For this review, take the finished solid that the model builds, in its own axes (mm). A direction names the side the tool comes from. Round coordinates to 2 decimals unless told otherwise and drop trailing zeros. Write each loop counter-clockwise with the first axis right and the second up, starting at its lowest first coordinate (ties: lowest second). Pieces come first, ordered by that corner, then holes. Notation, with made-up numbers: M 32.25,18 L 66.25,18 A4 cw 66.25,22 Z; hole C 64,-20.5 d5. An arc over 180 degrees is marked long. Answer in a Markdown table with one row per item.
```python
from build123d import *

# Parameters (mm, degrees)
SKETCH_1_W          = 50
SKETCH_1_H          = 20
EXTRUDE_1_DEPTH     = 2
SKETCH_2_R          = 3
EXTRUDE_2_DEPTH     = 2
EXTRUDE_START       = -2
SKETCH_3_R          = 3
EXTRUDE_3_DEPTH     = 2
SKETCH_4_R          = 1.5
CUT_EXTRUDE_1_DEPTH = 2


with BuildPart() as part:
    # 草图1 → 凸台-拉伸1 (new body)
    with BuildSketch(Plane(origin=(0, 0, 0), x_dir=(1, 0, 0), z_dir=(0, 1, 0))):
        Rectangle(SKETCH_1_W, SKETCH_1_H)
    extrude(amount=EXTRUDE_1_DEPTH)

    # 草图2 → 凸台-拉伸2 (add)
    with BuildSketch(Plane.ZY.offset(25)):
        with BuildLine():
            Line((-10, 2), (10, 2))
            Line((10, 2), (10, -18.1))
            ThreePointArc((10, -18.1), (7.100357134, -25.100357134), (0.1, -28))
            Line((0.1, -28), (-0.1, -28))
            ThreePointArc((-0.1, -28), (-7.100357134, -25.100357134), (-10, -18.1))
            Line((-10, -18.1), (-10, 2))
        make_face()
        with Locations((0, -18.1)):
            Circle(SKETCH_2_R, mode=Mode.SUBTRACT)
    extrude(amount=-EXTRUDE_2_DEPTH)

    # 草图3 → 凸台-拉伸3 (add)
    with BuildSketch(Plane(origin=(25, 0, 0), x_dir=(0, 0, -1), z_dir=(1, 0, 0)).offset(EXTRUDE_START)):
        with BuildLine():
            Line((-10, 2), (10, 2))
            Line((10, 2), (10, -18.1))
            ThreePointArc((10, -18.1), (7.100357134, -25.100357134), (0.1, -28))
            Line((0.1, -28), (-0.1, -28))
            ThreePointArc((-0.1, -28), (-7.100357134, -25.100357134), (-10, -18.1))
            Line((-10, -18.1), (-10, 2))
        make_face()
        with Locations(Location((0, -18.1, 0), (0, 0, 180))):
            Circle(SKETCH_3_R, mode=Mode.SUBTRACT)
    extrude(amount=EXTRUDE_3_DEPTH)

    # 草图4 → 切除-拉伸1 (cut)
    with BuildSketch(Plane(origin=(0, 2, 0), x_dir=(1, 0, 0), z_dir=(0, 1, 0))):
        with Locations(Location((0, 5, 0), (0, 0, 270))):
            Circle(SKETCH_4_R)
        with Locations(Location((5, 0, 0), (0, 0, 270))):
            Circle(SKETCH_4_R)
        with Locations(Location((0, -5, 0), (0, 0, 270))):
            Circle(SKETCH_4_R)
        with Locations(Location((-5, 0, 0), (0, 0, 270))):
            Circle(SKETCH_4_R)
    extrude(amount=-CUT_EXTRUDE_1_DEPTH, mode=Mode.SUBTRACT)


solid = part.part
```
Q1. Mouldability with a two-part tool opening along Z and no side actions: class faces 1 (the face through (25, -13, 0)), 2 (the face through (-24, -25, 7.2)), 3 (the face through (-3.513, 1.014, -0.195)) as +Z half, -Z half, draft (parallel to the pull), parting line (faces both ways), or undercut.
Found:
| item | result |
|---|---|
| face 1 | draft |
| face 2 | +Z half |
| face 3 | undercut |
Q2. Machinability: for faces 4 (the face through (0, 2, 0)), 5 (the face through (0, 0, 0)), which of the approach directions +Z, -Z, +X, -X, +Y, -Y give a long, thin tool a straight path to every point of the face, cutting with its end or side? Answer none if there is none.
Found:
| item | result |
|---|---|
| face 4 | +Z, -Z, +X, -X, +Y |
| face 5 | +Z, -Z, -Y |
Q3. Take a section at C-C (z = 6). State the section outline as (x, y) points, then the cut area to 3 significant figures.
Found:
| item | result |
|---|---|
| outline | M -25,-26.05 L -23,-26.05 L -23,0 L -1.12,0 L -1.12,2 L -25,2 Z; M 1.12,0 L 23,0 L 23,-26.05 L 25,-26.05 L 25,2 L 1.12,2 Z |
| area | 200 mm² |
Q4. For probe 1 along X at (y, z) = (1.1, 0); probe 2 along Z at (x, y) = (24.45, -18.1); probe 3 along X at (y, z) = (-13.75, -1), list the stretches that pass through material, from the lowest coordinate up.
Found:
| item | result |
|---|---|
| probe 1 | -25 to -6.5, -3.5 to 3.5, 6.5 to 25 |
| probe 2 | -10 to -3, 3 to 10 |
| probe 3 | -25 to -23, 23 to 25 |
Q5. Take a section at B-B (y = -2.25). State the section outline as (x, z) points.
Found:
| item | result |
|---|---|
| outline | M -25,-10 L -23,-10 L -23,10 L -25,10 Z; M 23,-10 L 25,-10 L 25,10 L 23,10 Z |
Q6. Take a section at D-D (x = 0). State the section outline as (y, z) points, then the cut area to 3 significant figures.
Found:
| item | result |
|---|---|
| outline | M 0,-10 L 2,-10 L 2,-6.5 L 0,-6.5 Z; M 0,-3.5 L 2,-3.5 L 2,3.5 L 0,3.5 Z; M 0,6.5 L 2,6.5 L 2,10 L 0,10 Z |
| area | 28.0 mm² |
Q7. Take a section at A-A (x = -5). State the section outline as (y, z) points, then the cut area to 3 significant figures.
Found:
| item | result |
|---|---|
| outline | M 0,-10 L 2,-10 L 2,-1.5 L 0,-1.5 Z; M 0,1.5 L 2,1.5 L 2,10 L 0,10 Z |
| area | 34.0 mm² |
Q8. Insertion check: P1, Ø5, axis at x = 0, z = -5, coming from the -Y side. The pin has a flat end and moves straight along its axis. Give the tip position at first contact, or say it passes through.
Found:
| item | result |
|---|---|
| P1 | y = 0 |
